from build123d import *

# Parameters (mm, degrees)
BOSS_EXTRUDE1_DEPTH = 8
BOSS_EXTRUDE2_DEPTH = 3


with BuildPart() as part:
    # Sketch1 → Boss-Extrude1 (new body)
    with BuildSketch(Plane.XY):
        with BuildLine():
            Line((70, 0), (70, 99))
            ThreePointArc((70, 99), (69.414213562, 100.414213562), (68, 101))
            Line((68, 101), (-68, 101))
            ThreePointArc((-68, 101), (-69.414213562, 100.414213562), (-70, 99))
            Line((-70, 99), (-70, 0))
            Line((-70, 0), (70, 0))
        make_face()
    extrude(amount=BOSS_EXTRUDE1_DEPTH)

    # Sketch2 → Boss-Extrude2 (add)
    with BuildSketch(Plane.XY.offset(8)):
        with BuildLine():
            Line((72, 0), (72, 99))
            ThreePointArc((72, 99), (70.828427125, 101.828427125), (68, 103))
            Line((68, 103), (-68, 103))
            ThreePointArc((-68, 103), (-70.828427125, 101.828427125), (-72, 99))
            Line((-72, 99), (-72, 0))
            Line((-72, 0), (72, 0))
        make_face()
    extrude(amount=-BOSS_EXTRUDE2_DEPTH)

    # Sketch3 → CSK for M4 Countersunk Flat Head Screw1 (revolve, cut)
    with BuildSketch(Plane(origin=(40, 10, 8), x_dir=(0, -1, 0), z_dir=(1, 0, 0))):
        Polygon((0, 0), (0, 8), (2.25, 8), (2.25, 3.45), (4.7, 1), (4.7, 0), align=None)
    csk_for_m4_countersunk_flat_head_screw1 = revolve(axis=Axis((40, 10, 14.35), (0, 0, -1)), mode=Mode.SUBTRACT)

    # Mirror1: CSK for M4 Countersunk Flat Head Screw1 across plane
    add(csk_for_m4_countersunk_flat_head_screw1.mirror(Plane(origin=(0, 0, 0), x_dir=(0, 0, 1), z_dir=(1, 0, 0))), mode=Mode.SUBTRACT)


solid = part.part
The listing builds one solid part. Answer for the finished solid, in the listing's coordinates (mm). A direction names the side the tool comes from. Give positions to 0.01 mm unless a question says otherwise; leave off trailing zeros. Write each loop counter-clockwise with the first axis right and the second up, starting at its lowest first coordinate (ties: lowest second). Pieces come first, ordered by that corner, then holes.
Item 1: Section A-A, the plane z = 3.25 is taken. Write down the section's boundary in (x, y).
Item 2: Flat-ended cylindrical pins translate along their axes: P1, Ø1, axis at y = 21, z = 2, coming from the -X side; P2, Ø7, axis at x = -40, y = 10, coming from the +Z side. Find the tip coordinate at first contact, or state that the pin passes through.
Item 3: Determine the mould class of faces 1 (the conical face through (42.13, 8.89, 4.7)), 2 (the flat face through (-1, 52, 8)), 3 (the flat face through (-1, 0, 4)) for opening direction Y: released by +Y, released by -Y, zero draft, split by the parting line, or undercut.
Item 4: Which of the six approach directions +Z, -Z, +X, -X, +Y, -Y give full straight-line access (tool end or side, diameter ignored) to faces 4 (the flat face through (70, 49, 2)), 5 (the flat face through (1, 101, 2)), 6 (the flat face through (-70, 50, 2)), 7 (the cylindrical face through (-44.17, 7.83, 7.51)), 8 (the flat face through (72, 49, 7))?
Item 5: Find the intervals of material crossed by line 1 along X through (y, z) = (10, 7.6); line 2 along X through (y, z) = (10, 2.7); line 3 along X through (y, z) = (61, 3.5), in increasing order.
Item 6: Section C-C, the plane x = 40 is taken. Write down the section's boundary in (y, z), plus the area to 3 significant figures.
Item 7: Section B-B, the plane y = 10 is taken. Write down the section's boundary in (x, z).
Item 8: Section D-D, the plane y = 42 is taken. Write down the section's boundary in (x, z), plus the area to 3 significant figures.
Completed:
1. outline: (-70, 0) - (70, 0) - (70, 99) arc R2 ccw to (68, 101) - (-68, 101) arc R2 ccw to (-70, 99) - close; hole circle Ø4.5 at (-40, 10); hole circle Ø4.5 at (40, 10)
2. P1: stops at x = -70
2. P2: stops at z = 5.8
3. face 1: undercut
3. face 2: zero draft
3. face 3: released by -Y
4. face 4: -Z, +X, +Y, -Y
4. face 5: -Z, +X, -X, +Y
4. face 6: -Z, -X, +Y, -Y
4. face 7: +Z
4. face 8: +Z, -Z, +X, +Y, -Y
5. line 1: x = -72 to -44.7, -35.3 to 35.3, 44.7 to 72
5. line 2: x = -70 to -42.25, -37.75 to 37.75, 42.25 to 70
5. line 3: x = -70 to 70
6. outline: (0, 0) - (7.75, 0) - (7.75, 4.55) - (5.3, 7) - (5.3, 8) - (0, 8) - close; (12.25, 0) - (101, 0) - (101, 5) - (103, 5) - (103, 8) - (14.7, 8) - (14.7, 7) - (12.25, 4.55) - close
6. area: 767 mm2
7. outline: (-72, 5) - (-70, 5) - (-70, 0) - (-42.25, 0) - (-42.25, 4.55) - (-44.7, 7) - (-44.7, 8) - (-72, 8) - close; (-37.75, 0) - (37.75, 0) - (37.75, 4.55) - (35.3, 7) - (35.3, 8) - (-35.3, 8) - (-35.3, 7) - (-37.75, 4.55) - close; (42.25, 0) - (70, 0) - (70, 5) - (72, 5) - (72, 8) - (44.7, 8) - (44.7, 7) - (42.25, 4.55) - close
8. outline: (-72, 5) - (-70, 5) - (-70, 0) - (70, 0) - (70, 5) - (72, 5) - (72, 8) - (-72, 8) - close
8. area: 1,130 mm2
